from build123d import *

# Parameters (mm, degrees)
SKETCH1_R           = 3.175
SKETCH1_R_2         = 3.81
BOSS_EXTRUDE1_DEPTH = 3.175


with BuildPart() as part:
    # Sketch1 → Boss-Extrude1 (new body, symmetric)
    with BuildSketch(Plane(origin=(0, 0, 0), x_dir=(1, 0, 0), z_dir=(0, 1, 0))):
        with BuildLine():
            Line((-228.6, 76.2), (228.6, 76.2))
            ThreePointArc((228.6, 76.2), (304.8, 0), (228.6, -76.2))
            Line((228.6, -76.2), (-228.6, -76.2))
            ThreePointArc((-228.6, -76.2), (-304.8, 0), (-228.6, 76.2))
        make_face()
        with Locations((-228.6, 0)):
            Circle(SKETCH1_R, mode=Mode.SUBTRACT)
        with Locations((-228.6, 50.8)):
            Circle(SKETCH1_R_2, mode=Mode.SUBTRACT)
        with Locations((-192.678975516, 35.921024484)):
            Circle(SKETCH1_R_2, mode=Mode.SUBTRACT)
        with Locations((-177.8, 0)):
            Circle(SKETCH1_R_2, mode=Mode.SUBTRACT)
        with Locations((-192.678975516, -35.921024484)):
            Circle(SKETCH1_R_2, mode=Mode.SUBTRACT)
        with Locations((-228.6, -50.8)):
            Circle(SKETCH1_R_2, mode=Mode.SUBTRACT)
        with Locations((-264.521024484, -35.921024484)):
            Circle(SKETCH1_R_2, mode=Mode.SUBTRACT)
        with Locations((-279.4, 0)):
            Circle(SKETCH1_R_2, mode=Mode.SUBTRACT)
        with Locations((-264.521024484, 35.921024484)):
            Circle(SKETCH1_R_2, mode=Mode.SUBTRACT)
        with Locations((228.6, 0)):
            Circle(SKETCH1_R, mode=Mode.SUBTRACT)
        with Locations((279.4, 0)):
            Circle(SKETCH1_R_2, mode=Mode.SUBTRACT)
        with Locations((264.521024484, -35.921024484)):
            Circle(SKETCH1_R_2, mode=Mode.SUBTRACT)
        with Locations((228.6, -50.8)):
            Circle(SKETCH1_R_2, mode=Mode.SUBTRACT)
        with Locations((192.678975516, -35.921024484)):
            Circle(SKETCH1_R_2, mode=Mode.SUBTRACT)
        with Locations((177.8, 0)):
            Circle(SKETCH1_R_2, mode=Mode.SUBTRACT)
        with Locations((192.678975516, 35.921024484)):
            Circle(SKETCH1_R_2, mode=Mode.SUBTRACT)
        with Locations((228.6, 50.8)):
            Circle(SKETCH1_R_2, mode=Mode.SUBTRACT)
        with Locations((264.521024484, 35.921024484)):
            Circle(SKETCH1_R_2, mode=Mode.SUBTRACT)
        with Locations((-127, 25.4)):
            Circle(SKETCH1_R_2, mode=Mode.SUBTRACT)
        with Locations((-76.2, -25.4)):
            Circle(SKETCH1_R_2, mode=Mode.SUBTRACT)
        with Locations((-127, -25.4)):
            Circle(SKETCH1_R_2, mode=Mode.SUBTRACT)
        with Locations((-76.2, 25.4)):
            Circle(SKETCH1_R_2, mode=Mode.SUBTRACT)
    extrude(amount=BOSS_EXTRUDE1_DEPTH, both=True)


solid = part.part
CAD build for the part. Positions are in the model's coordinates, mm. Coordinates: 2 decimals unless noted, no trailing zeros. Write each loop counter-clockwise with the first axis right and the second up, starting at its lowest first coordinate (ties: lowest second). Pieces come first, ordered by that corner, then holes. Notation, with made-up numbers: (-22, -36) - (-2, -36) arc R13 cw to (-2, -14) - close; hole circle Ø3 at (64.25, 24.25). An arc over 180 degrees is marked (long way). Use a Markdown table: item, result. Add a question column.
Item 1: Flat gauge pins, fed straight in: pin 1 (3 mm diameter, centred on y = 2.5, z = -42, fed in from -X); pin 2 (2 mm diameter, centred on y = -2, z = 39, fed in from +X). Where does each tip first touch, or does it go through?
Item 2: Band-saw the part on B-B, the plane z = 63.5. Give the cut face in (x, y) (3 decimals), and give its area (3 significant figures).
Item 3: Band-saw the part on A-A, the plane y = 1. Give the number of separate pieces and of enclosed holes in the cut face, and give its area (3 significant figures).
Item 4: Drill centre lines: L1, parallel to Z at x = 228.6, y = 1.5 (3 decimals); L2, parallel to Z at x = -127, y = -2; L3, parallel to X at y = 1, z = 3.5. Where is each one in solid material? Low to high. Write a range as from..to.
Numbers:
| question | item | result |
|---|---|---|
| 1 | pin 1 | x = -293.15 |
| 1 | pin 2 | x = 294.65 |
| 2 | outline | (-270.721, -3.175) - (270.721, -3.175) - (270.721, 3.175) - (-270.721, 3.175) - close |
| 2 | area | 3,440 mm2 |
| 3 | separate pieces | 1 |
| 3 | enclosed holes | 22 |
| 3 | area | 86,900 mm2 |
| 4 | L1 | -76.2..-54.61, -46.99..-3.175, 3.175..46.99, 54.61..76.2 |
| 4 | L2 | -76.2..-29.21, -21.59..21.59, 29.21..76.2 |
| 4 | L3 | -304.72..-280.91, -277.89..-179.31, -176.29..176.29, 179.31..277.89, 280.91..304.72 |
